```python
from build123d import *

# Parameters (mm, degrees)
F0_R          = 45.255389
F0_R_2        = 5.734106
F1_DEPTH      = 5
F2_R          = 45.255389
F2_W          = 27.738073
F2_H          = 40.435255
F3_DEPTH      = 100
F3_DEPTH_BACK = 25.4


with BuildPart() as f1:
    # F0 (on Front) → F1 (new body, symmetric)
    with BuildSketch(Plane.XZ):
        Circle(F0_R)
        Circle(F0_R_2, mode=Mode.SUBTRACT)
    extrude(amount=F1_DEPTH, both=True)

    # F2 (on face) → F3 (join, two sides)
    with BuildSketch(Plane.XZ.offset(5)) as f3_sk:
        Circle(F2_R)
        with Locations((0.834415, -2.516448)):
            Rectangle(F2_W, F2_H, mode=Mode.SUBTRACT)
    extrude(amount=F3_DEPTH)
    extrude(f3_sk.sketch, amount=-F3_DEPTH_BACK)


solid = f1.part
```
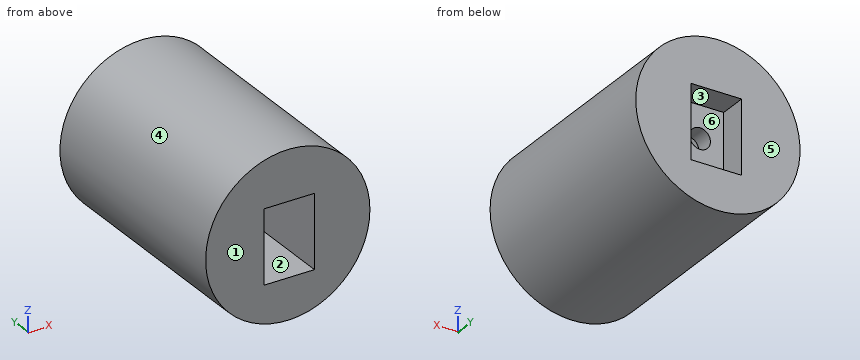
Design review of the part built by this model. Coordinates are the model's own, in mm. Face numbers are marked on the shaded views. A direction names the side the tool comes from. Give positions to 0.01 mm unless a question says otherwise; leave off trailing zeros. Loops run counter-clockwise (first coordinate to the right, second up) from the corner with the lowest first, then second, coordinate; pieces in that order, holes last. Notation, with made-up numbers: (4.25, 2.25) -> (33.25, 2.25) arc R4 ccw to (33.25, 6.25) -> close; hole circle Ø10 at (5.25, 21). An arc over 180 degrees is marked (long way). Write each question's results on one line, items separated by ' | '.
Q1. Take a section at A-A, the plane x = 0. Write out the cut boundary in (y, z), plus the area to 3 significant figures.
Reply:
outline: (-105, -45.26) -> (20.4, -45.26) -> (20.4, -22.73) -> (5, -22.73) -> (5, -5.73) -> (-5, -5.73) -> (-5, -22.73) -> (-105, -22.73) -> close; (-105, 17.7) -> (-5, 17.7) -> (-5, 5.73) -> (5, 5.73) -> (5, 17.7) -> (20.4, 17.7) -> (20.4, 45.26) -> (-105, 45.26) -> close | area: 6,570 mm²
Q2. The part is to be moulded in two halves that separate along X. For the marked faces 4, 5 and 6, say which applies: +X half, -X half, draft (parallel to the pull), parting line (faces both ways), or undercut.
Reply:
face 4: parting line | face 5: draft | face 6: undercut
Q3. Machinability: for the marked faces 1, 2 and 3, which of the approach directions +Z, -Z, +X, -X, +Y, -Y give a long, thin tool a straight path to every point of the face, cutting with its end or side? Answer none if there is none.
Reply:
face 1: +Z, -Z, +X, -X, -Y | face 2: -Y | face 3: +Y
Q4. Take a section at B-B, the plane z = 0. Write out the cut boundary in (x, y).
Reply:
outline: (-45.26, -105) -> (-13.03, -105) -> (-13.03, -5) -> (-5.73, -5) -> (-5.73, 5) -> (-13.03, 5) -> (-13.03, 20.4) -> (-45.26, 20.4) -> close; (5.73, -5) -> (14.7, -5) -> (14.7, -105) -> (45.26, -105) -> (45.26, 20.4) -> (14.7, 20.4) -> (14.7, 5) -> (5.73, 5) -> close
Q5. Wall thickness on L1, parallel to Z at x = 0, y = -1; L2, parallel to Y at x = 8, z = 5.5; L3, parallel to X at y = -53.5, z = 3: over which ranges is each line inside the solid? List them lowest first.
Reply:
L1: z = -45.26 to -5.73, 5.73 to 45.26 | L2: y = -5 to 5 | L3: x = -45.16 to -13.03, 14.7 to 45.16
Q6. For pin 1 Ø22 at (x, z) = (-2, 5.5) entering from +Y; pin 2 Ø10 at (y, z) = (-84, 17.5) entering from -X; pin 3 Ø12 at (y, z) = (-5.5, 27) entering from +X, all flat-tipped, find the tip position at first contact; note any pin that passes through.
Reply:
pin 1: stops at y = 5 | pin 2: stops at x = -43.49 | pin 3: stops at x = 40.09
Q7. Take a section at C-C, the plane y = -41.5. Write out the cut boundary in (x, z), plus the area to 3 significant figures.
Reply:
outline: circle Ø90.51 at (0, 0); hole (-13.03, -22.73) -> (14.7, -22.73) -> (14.7, 17.7) -> (-13.03, 17.7) -> close | area: 5,310 mm²
Q8. Take a section at D-D, the plane z = -31. Write out the cut boundary in (x, y).
Reply:
outline: (-32.97, -105) -> (32.97, -105) -> (32.97, 20.4) -> (-32.97, 20.4) -> close
